Autodesk Inventor part; units mm, degrees
ref_plane "YZ Plane" through (0, 0, 0) normal (1, 0, 0) x (0, 1, 0)
ref_plane "XZ Plane" through (0, 0, 0) normal (0, 1, 0) x (-1, 0, 0)
ref_plane "XY Plane" through (0, 0, 0) normal (0, 0, 1) x (1, 0, 0)
sketch "Sketch1" plane through (0, 0, 0) normal (1, 0, 0) x (0, 1, 0)
  line L0 (0, 0) -> (48.26, 0)
  line L1 (48.26, 0) -> (48.26, -25.4)
  line L2 (48.26, -25.4) -> (0, -25.4)
  line L3 (0, -25.4) -> (0, 0)
  line L4 (0, 0) -> (24.13, 0) construction
  line L5 (24.13, 0) -> (24.13, -25.4) construction
  line L6 (24.13, -25.4) -> (0, -25.4) construction
  line L7 (0, -25.4) -> (0, 0) construction
  line L8 (24.13, 0) -> (0, -25.4) construction
  line L9 (0, 0) -> (24.13, -25.4) construction
  line L10 (24.13, 0) -> (48.26, -25.4) construction
  line L11 (48.26, 0) -> (24.13, -25.4) construction
  circle A0 centre (12.065, -12.7) radius 3.175
  circle A1 centre (36.195, -12.7) radius 3.175
  dimension "d0" = 48.26
  dimension "d1" = 25.4
  dimension "d2" = 24.13
  dimension "d3" = 25.4
  dimension "d32" = 6.35
  dimension "d33" = 6.35
extrude "Extrusion1" add sketch "Sketch1" against normal blind 7.9375
sketch "Sketch2" plane through (0, 48.26, 0) normal (0, 1, 0) x (1, 0, 0)
  line L0 (0, 0) -> (-25.4, 0)
  line L1 (-25.4, 0) -> (-25.4, 25.4)
  line L2 (-25.4, 25.4) -> (0, 25.4)
  line L3 (0, 25.4) -> (0, 0)
  line L4 (0, 0) -> (-7.9375, 0) construction
  line L5 (-25.4, 25.4) -> (0, 0) construction
  line L6 (0, 0) -> (0, 25.4) construction
  line L7 (0, 25.4) -> (-25.4, 0) construction
  circle A0 centre (-12.7, 12.7) radius 3.175
  dimension "d8" = 25.4
  dimension "d9" = 25.4
  dimension "d34" = 6.35
extrude "Extrusion2" add sketch "Sketch2" against normal blind 7.9375
sketch "Sketch5" plane through (-7.9375, 0, 0) normal (0, 0, 1) x (1, 0, 0)
  line L0 (7.9375, 0) -> (7.9375, 48.26)
  line L1 (7.9375, 0) -> (-17.4625, 0)
  line L2 (-17.4625, 0) -> (-17.4625, 7.9375)
  line L3 (-17.4625, 7.9375) -> (7.9375, 7.9375)
  line L4 (7.9375, 7.9375) -> (7.9375, 0)
  dimension "d19" = 25.4
  dimension "d20" = 7.9375
extrude "Extrusion3" add sketch "Sketch5" against normal blind 25.4
sketch "Sketch6" plane through (0, 0, -25.4) normal (0, -1, 0) x (1, 0, 0)
  line L0 (-7.9375, 25.4) -> (-25.4, 25.4) construction
  line L1 (0, 0) -> (-25.4, 0) construction
  line L2 (-25.4, 25.4) -> (0, 0) construction
  line L3 (0, 0) -> (0, 25.4) construction
  line L4 (-25.4, 0) -> (0, 25.4) construction
  circle A0 centre (-12.7, 12.7) radius 3.175
  dimension "d35" = 6.35
sketch "Sketch7" plane through (0, 0, 0) normal (1, 0, 0) x (0, 0, -1)
  line L0 (0, 0) -> (25.4, 0) construction
  line L1 (25.4, 0) -> (25.4, 24.13) construction
  line L2 (25.4, 24.13) -> (0, 24.13) construction
  line L3 (0, 24.13) -> (0, 0) construction
  line L4 (0, 0) -> (25.4, 24.13) construction
  line L5 (0, 24.13) -> (25.4, 0) construction
  line L6 (0, 24.13) -> (25.4, 48.26) construction
  line L7 (25.4, 48.26) -> (0, 48.26) construction
  line L8 (25.4, 24.13) -> (0, 48.26) construction
  circle A0 centre (12.7, 12.065) radius 9.525
  circle A1 centre (12.7, 36.195) radius 9.525
  dimension "d26" = 25.4
  dimension "d27" = 24.13
  dimension "d28" = 19.05
  dimension "d29" = 19.05
extrude "Extrusion5" cut sketch "Sketch7" against normal blind 3.175
extrude "Extrusion6" cut sketch "Sketch6" against normal blind 7.9375
sketch "Sketch8" plane through (0, 0, -25.4) normal (0, -1, 0) x (1, 0, 0)
  line L0 (-7.9375, 25.4) -> (-25.4, 25.4) construction
  line L1 (0, 0) -> (-25.4, 0) construction
  line L2 (-25.4, 25.4) -> (0, 0) construction
  line L3 (0, 0) -> (0, 25.4) construction
  line L4 (-25.4, 25.4) -> (-25.4, 0) construction
  line L5 (0, 25.4) -> (-25.4, 0) construction
  circle A0 centre (-12.7, 12.7) radius 9.525
  dimension "d38" = 19.05
extrude "Extrusion7" cut sketch "Sketch8" against normal blind 3.175
sketch "Sketch9" plane through (0, 48.26, 0) normal (0, 1, 0) x (1, 0, 0)
  line L0 (-25.4, 25.4) -> (-7.9375, 25.4) construction
  line L1 (0, 0) -> (-25.4, 25.4) construction
  line L2 (-7.9375, 0) -> (-25.4, 0) construction
  line L3 (0, 25.4) -> (-25.4, 25.4) construction
  line L4 (-25.4, 0) -> (0, 25.4) construction
  circle A0 centre (-12.7, 12.7) radius 9.525
  dimension "d41" = 19.05
extrude "Extrusion8" cut sketch "Sketch9" against normal blind 3.175
properties part number "MountingBracket_Double"
Part model, mm, in its own coordinate system. A direction names the side the tool comes from. Give positions to 0.01 mm unless a question says otherwise; leave off trailing zeros. Order: outer loops, then holes, each group sorted by start corner. A loop starts at its lowest first (then second) coordinate and runs counter-clockwise, first axis right, second up. Notation, with made-up numbers: (-38, -23) - (-31, -23) arc R18 cw to (-31, -17) - close; hole circle Ø4 at (-23, 42). An arc over 180 degrees is marked (long way). Use a Markdown table: item, result.
1) Saw through at B-B on x = -23.5. List the corners of the cut face in (y, z), plus the area to 3 significant figures.
Checked values:
| item | result |
|---|---|
| outline | (0, -25.4) - (7.94, -25.4) - (7.94, 0) - (0, 0) - close; (40.32, -25.4) - (48.26, -25.4) - (48.26, 0) - (40.32, 0) - close |
| area | 403 mm² |
2) Saw through at C-C on y = 34.5. List the corners of the cut face in (x, z) (1 decimal).
Checked values:
| item | result |
|---|---|
| outline | (-7.9, -25.4) - (0, -25.4) - (0, -22.1) - (-3.2, -22.1) - (-3.2, -15.4) - (-7.9, -15.4) - close; (-7.9, -10) - (-3.2, -10) - (-3.2, -3.3) - (0, -3.3) - (0, 0) - (-7.9, 0) - close |
3) Two-plate mould, pull along X, no slides. Class faces 1 (the flat face through (-3.175, 32, -13)), 2 (the flat face through (-7, 24, -25.4)), 3 (the cylindrical face through (-20.259, 46.695, -6.904)): +X half, -X half, draft (parallel to the pull), parting line (faces both ways), or undercut.
Checked values:
| item | result |
|---|---|
| face 1 | +X half |
| face 2 | draft |
| face 3 | undercut |
4) Flat gauge pins, fed straight in: P1, Ø12, axis at y = 20.5, z = -13, coming from the -X side; P2, Ø5.5, axis at y = 34, z = -12, coming from the +X side (3 decimals); P3, Ø7.5, axis at x = -12.7, z = -12.7, coming from the -Y side (3 decimals). Where does each tip first touch, or does it go through?
Checked values:
| item | result |
|---|---|
| P1 | x = -7.94 |
| P2 | x = -3.175 |
| P3 | y = 3.175 |
5) Saw through at D-D on z = -17.25. List the corners of the cut face in (x, y) (1 decimal), plus the area to 3 significant figures.
Checked values:
| item | result |
|---|---|
| outline | (-25.4, 0) - (-21.1, 0) - (-21.1, 3.2) - (-4.3, 3.2) - (-4.3, 0) - (0, 0) - (0, 3.7) - (-3.2, 3.7) - (-3.2, 20.4) - (0, 20.4) - (0, 27.8) - (-3.2, 27.8) - (-3.2, 44.6) - (0, 44.6) - (0, 48.3) - (-4.3, 48.3) - (-4.3, 45.1) - (-21.1, 45.1) - (-21.1, 48.3) - (-25.4, 48.3) - (-25.4, 40.3) - (-7.9, 40.3) - (-7.9, 7.9) - (-25.4, 7.9) - close |
| area | 448 mm² |
6) Saw through at A-A on x = -12.7. List the corners of the cut face in (y, z) (1 decimal), plus the area to 3 significant figures.
Checked values:
| item | result |
|---|---|
| outline | (0, -25.4) - (7.9, -25.4) - (7.9, -15.9) - (3.2, -15.9) - (3.2, -22.2) - (0, -22.2) - close; (0, -3.2) - (3.2, -3.2) - (3.2, -9.5) - (7.9, -9.5) - (7.9, 0) - (0, 0) - close; (40.3, -25.4) - (48.3, -25.4) - (48.3, -22.2) - (45.1, -22.2) - (45.1, -15.9) - (40.3, -15.9) - close; (40.3, -9.5) - (45.1, -9.5) - (45.1, -3.2) - (48.3, -3.2) - (48.3, 0) - (40.3, 0) - close |
| area | 222 mm² |
7) Probe L1, parallel to Y at x = -1.9, z = -12.7; L2, parallel to Y at x = -19.5, z = -4.25; L3, parallel to Z at x = -12.7, y = 5 (3 decimals). List the from-to ranges inside material, lowest first. Write a range as from..to.
Checked values:
| item | result |
|---|---|
| L1 | 0..2.54, 21.59..26.67, 45.72..48.26 |
| L2 | 0..7.94, 40.32..48.26 |
| L3 | -25.4..-15.875, -9.525..0 |
8) 3-axis set-ups, long thin cutter, end or side, ignore diameter. For faces 4 (the cylindrical face through (-1.57, 18.5, -5.68)), 5 (the flat face through (-7.938, 24, -13)), 6 (the flat face through (-4, 0, -7)): which of +Z, -Z, +X, -X, +Y, -Y reach the whole face in a straight line?
Checked values:
| item | result |
|---|---|
| face 4 | +X |
| face 5 | +Z, -Z, -X |
| face 6 | +Z, -Z, +X, -X, -Y |
